The model under review builds one solid part; all positions refer to its coordinate system, in mm. A direction names the side the tool comes from. Round coordinates to 2 decimals unless told otherwise and drop trailing zeros. Loops run counter-clockwise (first coordinate to the right, second up) from the corner with the lowest first, then second, coordinate; pieces in that order, holes last. Notation, with made-up numbers: (70, -35.75) -> (127, -35.75) arc R21 ccw to (127, -13.75) -> close; hole circle Ø8 at (-37, 32). An arc over 180 degrees is marked (long way). Use a Markdown table: item, result. Add a question column.
1) Consider section C-C on y = 2. State how many separate pieces and enclosed holes the cut face has, plus the area to 3 significant figures.
2) Consider section A-A on z = -60. Give the boundary of the cut face in (x, y).
3) Wall thickness on probe 1 along Y at (x, z) = (42.5, -51); probe 2 along X at (y, z) = (0, 11); probe 3 along X at (y, z) = (-19, -28.5): over which ranges is each line inside the solid? List them lowest first.
4) Consider section B-B on x = -43.5. Give the boundary of the cut face in (y, z), plus the area to 3 significant figures.
5) Insertion check: pin 1 (2 mm diameter, centred on x = 8, y = -13, fed in from +Z); pin 2 (12 mm diameter, centred on x = -8.5, y = 19, fed in from +Z); pin 3 (9 mm diameter, centred on x = -2.5, y = 4.5, fed in from +Z); pin 4 (10 mm diameter, centred on y = -2.5, z = -34.5, fed in from -X). Each pin has a flat end and moves straight along its axis. Give the tip position at first contact, or say it passes through.
6) For faces 1 (the flat face through (40, -9, -36)), 2 (the flat face through (0, 0, 0)), 3 (the flat face through (-44, 1, 0)), 4 (the flat face through (-1, -40, -14)), 5 (the flat face through (43, 1, 0)), list the 3-axis set-ups (+Z, -Z, +X, -X, +Y, -Y) from which the entire face can be reached by the end or side of a thin tool; tool diameter is ignored.
7) Mouldability with a two-part tool opening along Y and no side actions: class faces 6 (the flat face through (1, 40, -14)), 7 (the cylindrical face through (50.14, -3.47, -65.62)), 8 (the flat face through (-60, 9, -34)) as released by +Y, released by -Y, zero draft, split by the parting line, or undercut.
from build123d import *

# Parameters (mm, degrees)
F0_R     = 30
F0_R_2   = 15
F1_DEPTH = 90
F2_R     = 16
F3_DEPTH = 120
F4_W     = 80
F4_H     = 35
F4_H_2   = 40
F5_DEPTH = 250


with BuildPart() as f1:
    # F0 (on Top) → F1 (new body)
    with BuildSketch(Plane.XY):
        with BuildLine():
            ThreePointArc((0, -40), (-40, 0), (0, 40))
            Line((0, 40), (-60, 40))
            Line((-60, 40), (-60, -40))
            Line((-60, -40), (0, -40))
        make_face()
        with BuildLine():
            ThreePointArc((0, -40), (28.284271, -28.284271), (40, 0))
            ThreePointArc((40, 0), (28.284271, 28.284271), (0, 40))
            ThreePointArc((0, 40), (-40, 0), (0, -40))
        make_face()
        Circle(F0_R, mode=Mode.SUBTRACT)
        Circle(F0_R)
        Circle(F0_R_2, mode=Mode.SUBTRACT)
        Circle(F0_R_2)
        with BuildLine():
            ThreePointArc((0, 40), (28.284271, 28.284271), (40, 0))
            ThreePointArc((40, 0), (28.284271, -28.284271), (0, -40))
            Line((0, -40), (60, -40))
            Line((60, -40), (60, 40))
            Line((60, 40), (0, 40))
        make_face()
    extrude(amount=-F1_DEPTH)

    # F2 (on face) → F3 (cut)
    with BuildSketch(Plane.YZ.offset(60)):
        with Locations((0, -50)):
            Circle(F2_R)
        with BuildLine():
            ThreePointArc((0, -90), (-28.284271, -78.284271), (-40, -50))
            Line((-40, -50), (-40, -90))
            Line((-40, -90), (0, -90))
        make_face()
        with BuildLine():
            Line((40, -90), (40, -50))
            ThreePointArc((40, -50), (28.284271, -78.284271), (0, -90))
            Line((0, -90), (40, -90))
        make_face()
    extrude(amount=-F3_DEPTH, mode=Mode.SUBTRACT)

    # F4 (on face) → F5 (cut)
    with BuildSketch(Plane.XZ.offset(40)):
        with Locations((0, -32.5)):
            Rectangle(F4_W, F4_H)
        with Locations((0, -70)):
            Rectangle(F4_W, F4_H_2)
    extrude(amount=-F5_DEPTH, mode=Mode.SUBTRACT)

    # F6 (on Front) → F7 (revolve)
    with BuildSketch(Plane.XZ):
        Polygon((-40, 0), (-15, 0), (-30, 5), (-30, 20), (-40, 20), align=None)
    revolve(axis=Axis((0, 0, 23.827048), (0, 0, 1)))


solid = f1.part
Result set:
| question | item | result |
|---|---|---|
| 1 | separate pieces | 3 |
| 1 | enclosed holes | 0 |
| 1 | area | 4,000 mm2 |
| 2 | outline | (-60, -38.73) -> (-40, -38.73) -> (-40, -12.49) -> (-60, -12.49) -> close; (-60, 12.49) -> (-40, 12.49) -> (-40, 38.73) -> (-60, 38.73) -> close; (40, -38.73) -> (60, -38.73) -> (60, -12.49) -> (40, -12.49) -> close; (40, 12.49) -> (60, 12.49) -> (60, 38.73) -> (40, 38.73) -> close |
| 3 | probe 1 | -39.99 to -15.97, 15.97 to 39.99 |
| 3 | probe 2 | -40 to -30, 30 to 40 |
| 3 | probe 3 | -60 to -40, 40 to 60 |
| 4 | outline | (-40, -50) arc R40 ccw to (0, -90) arc R40 ccw to (40, -50) -> (40, 0) -> (-40, 0) -> close; hole circle Ø32 at (0, -50) |
| 4 | area | 5,710 mm2 |
| 5 | pin 1 | z = 0.42 |
| 5 | pin 2 | z = 3.94 |
| 5 | pin 3 | z = 0 |
| 5 | pin 4 | x = -60 |
| 6 | face 1 | -Z, +Y, -Y |
| 6 | face 2 | +Z |
| 6 | face 3 | +Z, -X |
| 6 | face 4 | +Z, -Z, +X, -X, -Y |
| 6 | face 5 | +Z, +X |
| 7 | face 6 | released by +Y |
| 7 | face 7 | undercut |
| 7 | face 8 | zero draft |
